from build123d import *

# Parameters (mm, degrees)
F1_DEPTH = 38.1
F2_R     = 3.175
F3_DEPTH = 38.1
F4_R     = 6.35
F5_DEPTH = 12.7
F6_R     = 9.652


with BuildPart() as f1:
    # F0 (on Front) → F1 (new body)
    with BuildSketch(Plane.XZ):
        Polygon((-27.85063, -5.873353), (16.251101, -5.847953), (16.251101, 13.202047), (-28.198899, 13.202047), (-28.198899, 8.426847), (-7.198899, 8.426847), (-7.198899, -1.098153), (-27.85063, -1.098153), align=None)
    extrude(amount=F1_DEPTH)

    # F2 (on face) → F3 (cut)
    with BuildSketch(Plane.XY.offset(13.202047)):
        with Locations((-18.673899, -28.575)):
            Circle(F2_R)
        with Locations((-18.673899, -9.525)):
            Circle(F2_R)
    extrude(amount=-F3_DEPTH, mode=Mode.SUBTRACT)

    # F4 (on face) → F5 (cut)
    with BuildSketch(Plane.YZ.offset(16.251101)):
        with Locations((-19.05, 3.426872)):
            Circle(F4_R)
    extrude(amount=-F5_DEPTH, mode=Mode.SUBTRACT)

    # F6
    f6_edges = [f1.edges().sort_by_distance(p)[0] for p in [
        (-28.198899, -38.1, 10.814447),
        (-28.198899, 0, 10.814447),
        (-27.85063, 0, -3.485753),
        (-27.85063, -38.1, -3.485753),
        (-7.198899, -38.1, 3.664347),
        (-7.198899, 0, 3.664347),
    ]]
    fillet(f6_edges, radius=F6_R)


solid = f1.part
For this review, take the finished solid that the model builds, in its own axes (mm). A direction names the side the tool comes from. Round coordinates to 2 decimals unless told otherwise and drop trailing zeros. Order: outer loops, then holes, each group sorted by start corner. A loop starts at its lowest first (then second) coordinate and runs counter-clockwise, first axis right, second up. Notation, with made-up numbers: (69, 34.5) -> (81, 34.5) arc R22 ccw to (81, 56.5) -> close; hole circle Ø4 at (-24, 29). An arc over 180 degrees is marked (long way). Write item = value, one per line. Start each with the question number.
1) Take a section at D-D on y = -19.05. State the section outline as (x, z) points.
2) Take a section at B-B on z = -4. State the section outline as (x, y) points (3 decimals).
3) Insertion check: pin 1 (10 mm diameter, centred on x = -20.5, z = 2.5, fed in from +Y); pin 2 (5.5 mm diameter, centred on x = -18.67, y = -9.52, fed in from -Z); pin 3 (7.5 mm diameter, centred on x = -18.67, y = -28.58, fed in from -Z); pin 4 (5.5 mm diameter, centred on y = -17, z = -2.5, fed in from -X). Each pin has a flat end and moves straight along its axis. Give the tip position at first contact, or say it passes through.
4) Tool access review of faces 4 (the face through (-7.199, -19, 4)), 5 (the face through (3.551, -19, 4)), 6 (the face through (-25.098, -2.902, -3.519)): name each direction out of +Z, -Z, +X, -X, +Y, -Y from which nothing blocks a thin tool from reaching the whole face with its end or side.
5) Take a section at C-C on y = -8. State the section outline as (x, z) points, plus the area to 3 significant figures.
6) To check wall thickness, follow line 1 (Y direction, x = -20.5, z = -3.5); line 2 (Y direction, x = -17.5, z = -1.25); line 3 (X direction, y = -18, z = 2.25). State the ranges of each line that lie inside material, in increasing order. Write a range as from..to.
7) The part is to be moulded in two halves that separate along Y. For faces 1 (the face through (9.99, -24.089, -0.437)), 2 (the face through (-6, -19, 13.202)), 3 (the face through (-25.098, -35.198, -3.519)), say which applies: +Y half, -Y half, draft (parallel to the pull), parting line (faces both ways), or undercut.
8) Take a section at A-A on x = -16.5. State the section outline as (y, z) points, plus the area to 3 significant figures.
Verdict:
q1.outline = (-28.2, 8.43) -> (-7.2, 8.43) -> (-7.2, -1.1) -> (-27.85, -1.1) -> (-27.85, -5.87) -> (16.25, -5.85) -> (16.25, -2.92) -> (3.55, -2.92) -> (3.55, 9.78) -> (16.25, 9.78) -> (16.25, 13.2) -> (-28.2, 13.2) -> close
q2.outline = (-27.851, -28.448) arc R9.652 ccw to (-18.199, -38.1) -> (16.251, -38.1) -> (16.251, 0) -> (-18.199, 0) arc R9.652 ccw to (-27.851, -9.652) -> close; hole circle Ø6.35 at (-18.674, -28.575); hole circle Ø6.35 at (-18.674, -9.525)
q3.pin_1 = 0
q3.pin_2 = through
q3.pin_3 = -5.87
q3.pin_4 = -27.85
q4.face_4 = -X, +Y, -Y
q4.face_5 = +X
q4.face_6 = -Z, -X, +Y
q5.outline = (-28.06, 8.43) -> (-21.46, 8.43) -> (-21.46, 13.2) -> (-28.06, 13.2) -> close; (-27.71, -5.87) -> (-21.46, -5.87) -> (-21.46, -1.1) -> (-27.71, -1.1) -> close; (-15.89, -5.87) -> (16.25, -5.85) -> (16.25, 13.2) -> (-15.89, 13.2) -> (-15.89, 8.43) -> (-7.06, 8.43) -> (-7.06, -1.1) -> (-15.89, -1.1) -> close
q5.area = 590 mm2
q6.line_1 = -37.82..-31.17, -25.98..-12.12, -6.93..-0.28
q6.line_2 = -38.1..-31.53, -25.62..-12.48, -6.57..0
q6.line_3 = -7.2..3.55
q7.face_1 = undercut
q7.face_2 = draft
q7.face_3 = -Y half
q8.outline = (-38.1, -5.87) -> (-30.89, -5.87) -> (-30.89, -1.1) -> (-38.1, -1.1) -> close; (-38.1, 8.43) -> (-30.89, 8.43) -> (-30.89, 13.2) -> (-38.1, 13.2) -> close; (-26.26, -5.87) -> (-11.84, -5.87) -> (-11.84, -1.1) -> (-26.26, -1.1) -> close; (-26.26, 8.43) -> (-11.84, 8.43) -> (-11.84, 13.2) -> (-26.26, 13.2) -> close; (-7.21, -5.87) -> (0, -5.87) -> (0, -1.1) -> (-7.21, -1.1) -> close; (-7.21, 8.43) -> (0, 8.43) -> (0, 13.2) -> (-7.21, 13.2) -> close
q8.area = 275 mm2
